Geometry: final body of the model. Coordinates: model frame, mm. A direction names the side the tool comes from. Round coordinates to 2 decimals unless told otherwise and drop trailing zeros. Write each loop counter-clockwise with the first axis right and the second up, starting at its lowest first coordinate (ties: lowest second). Pieces come first, ordered by that corner, then holes. Notation, with made-up numbers: (48.5, 27) - (94.5, 27) arc R14 cw to (94.5, 51) - close; hole circle Ø11 at (9.5, -5). An arc over 180 degrees is marked (long way). Write each question's results on one line, items separated by ' | '.
from build123d import *

# Parameters (mm, degrees)
CROQUIS1_R              = 1.5875
SALIENTE_EXTRUIR1_DEPTH = 3.175
CROQUIS2_R              = 1.5875
CORTAR_EXTRUIR1_DEPTH   = 3.175
CROQUIS3_W              = 10
CROQUIS3_H              = 4.7625
SALIENTE_EXTRUIR2_DEPTH = 3.175


with BuildPart() as part:
    # Croquis1 → Saliente-Extruir1 (new body)
    with BuildSketch(Plane(origin=(0, 0, 0), x_dir=(1, 0, 0), z_dir=(0, 1, 0))):
        with BuildLine():
            Line((8.713785816, 43.568929081), (0, 0))
            Line((0, 0), (60, 0))
            Line((60, 0), (51.286214184, 43.568929081))
            ThreePointArc((51.286214184, 43.568929081), (48.513480023, 48.186737131), (43.441568778, 50))
            Line((43.441568778, 50), (16.558431222, 50))
            ThreePointArc((16.558431222, 50), (11.486519977, 48.186737131), (8.713785816, 43.568929081))
        make_face()
        with Locations((39.75, 14)):
            Circle(CROQUIS1_R, mode=Mode.SUBTRACT)
        with Locations((20.25, 14)):
            Circle(CROQUIS1_R, mode=Mode.SUBTRACT)
        with Locations((24.75, 44)):
            Circle(CROQUIS1_R, mode=Mode.SUBTRACT)
        with Locations((35.25, 44)):
            Circle(CROQUIS1_R, mode=Mode.SUBTRACT)
    extrude(amount=SALIENTE_EXTRUIR1_DEPTH)

    # Croquis2 → Cortar-Extruir1 (cut)
    with BuildSketch(Plane(origin=(0, 3.175, 0), x_dir=(1, 0, 0), z_dir=(0, 1, 0))):
        with Locations((30, 35)):
            Circle(CROQUIS2_R)
        with Locations((6.099019514, 5)):
            Circle(CROQUIS2_R)
        with Locations((53.900980486, 5)):
            Circle(CROQUIS2_R)
        with BuildLine():
            Line((53.900980486, 0), (60, 0))
            Line((60, 0), (58.803883865, 5.980580676))
            ThreePointArc((58.803883865, 5.980580676), (57.767691193, 1.830055472), (53.900980486, 0))
        make_face()
        with BuildLine():
            Line((1.196116135, 5.980580676), (0, 0))
            Line((0, 0), (6.099019514, 0))
            ThreePointArc((6.099019514, 0), (2.232308807, 1.830055472), (1.196116135, 5.980580676))
        make_face()
    extrude(amount=-CORTAR_EXTRUIR1_DEPTH, mode=Mode.SUBTRACT)

    # Croquis3 → Saliente-Extruir2 (add)
    with BuildSketch(Plane(origin=(0, 3.175, 0), x_dir=(1, 0, 0), z_dir=(0, 1, 0))):
        with Locations((20, -2.38125)):
            Rectangle(CROQUIS3_W, CROQUIS3_H)
        with Locations((40, -2.38125)):
            Rectangle(CROQUIS3_W, CROQUIS3_H)
    extrude(amount=-SALIENTE_EXTRUIR2_DEPTH)


solid = part.part
Q1. Mould query, pull axis Z, two halves, no side actions, for faces 1 (the cylindrical face through (52.315, 1.61, -5.07)), 2 (the flat face through (30, 0, -23)), 3 (the cylindrical face through (11.5, 1.6, -48.2)), 4 (the flat face through (20, 2, 4.762)). Classes: pulls with the +Z half, pulls with the -Z half, needs draft (parallel to the pull), parting line crosses it, or undercut.
Answer block:
face 1: undercut | face 2: needs draft | face 3: pulls with the -Z half | face 4: pulls with the +Z half
Q2. Section query A-A, the plane x = 20.25. Return loops of the section in (y, z) (1 decimal), plus the area to 3 significant figures.
Answer block:
outline: (0, -50) - (3.2, -50) - (3.2, -15.6) - (0, -15.6) - close; (0, -12.4) - (3.2, -12.4) - (3.2, 4.8) - (0, 4.8) - close | area: 164 mm2
Q3. Section query D-D, the plane z = -5. Return loops of the section in (x, y) (3 decimals).
Answer block:
outline: (1.099, 0) - (4.512, 0) - (4.512, 3.175) - (1.099, 3.175) - close; (7.687, 0) - (52.313, 0) - (52.313, 3.175) - (7.687, 3.175) - close; (55.488, 0) - (58.901, 0) - (58.901, 3.175) - (55.488, 3.175) - close
Q4. Section query B-B, the plane z = -35. Return loops of the section in (x, y) (1 decimal).
Answer block:
outline: (7, 0) - (28.4, 0) - (28.4, 3.2) - (7, 3.2) - close; (31.6, 0) - (53, 0) - (53, 3.2) - (31.6, 3.2) - close
Q5. Section query C-C, the plane y = 0.55. Give the number of separate pieces and of enclosed holes in the cut face, plus the area to 3 significant figures.
Answer block:
separate pieces: 1 | enclosed holes: 7 | area: 2,510 mm2
Q6. Access query for faces 5 (the flat face through (15, 2, 2)), 6 (the flat face through (30, 2, 0)), 7 (the flat face through (30, 3.175, -23)), 8 (the flat face through (5, 2, -25)), 9 (the flat face through (49, 2, 0)). Directions: +Z, -Z, +X, -X, +Y, -Y. A direction counts if a zero-diameter tool reaches every point of the face in a straight line with its end or side. Return the directions, or none.
Answer block:
face 5: +Z, -X, +Y, -Y | face 6: +Z, +Y, -Y | face 7: +Z, -Z, +X, -X, +Y | face 8: -Z, -X, +Y, -Y | face 9: +Z, +X, +Y, -Y
Q7. Ray query, line 1 along X through (y, z) = (2.3, -5); line 2 along Z through (x, y) = (39.75, 0.85); line 3 along X through (y, z) = (1.05, -4.5). Return the intervals inside material, ascending.
Answer block:
line 1: 1.1 to 4.51, 7.69 to 52.31, 55.49 to 58.9 | line 2: -50 to -15.59, -12.41 to 4.76 | line 3: 1.12 to 4.59, 7.61 to 52.39, 55.41 to 58.88
Q8. Pin query (flat end, axial travel): pin 1 (1 mm diameter, centred on x = 50, y = 2, fed in from +Z); pin 2 (1 mm diameter, centred on y = 1, z = 3, fed in from +X); pin 3 (1 mm diameter, centred on y = 1, z = -3.5, fed in from -X). Return the tip coordinate at first contact, or that it passes through.
Answer block:
pin 1: z = 0 | pin 2: x = 45 | pin 3: x = 1.2
